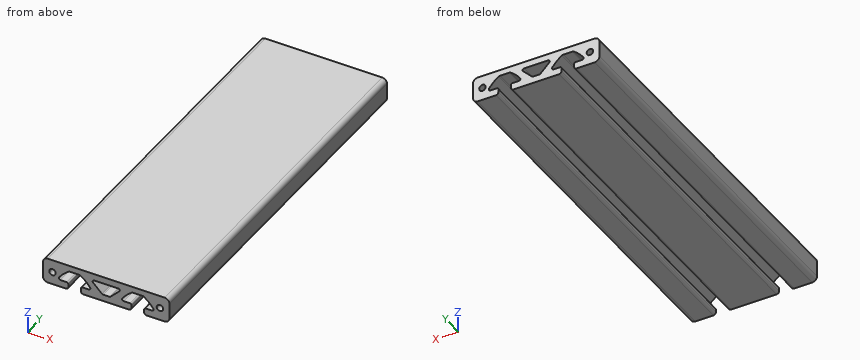
Autodesk Inventor part; units mm, degrees
ref_plane "Start Plane" through (0, 0, 0) normal (0, 1, 0) x (-1, 0, 0)
ref_plane "End Plane" through (0, 240, 0) normal (0, 1, 0) x (-1, 0, 0)
ref_plane "YZ Plane" through (0, 0, 0) normal (1, 0, 0) x (0, 1, 0)
ref_plane "Start Plane" through (0, 0, 0) normal (0, 1, 0) x (-1, 0, 0)
ref_plane "End Plane" through (0, 240, 0) normal (0, 1, 0) x (-1, 0, 0)
sketch "Sketch1" plane through (0, 0, 0) normal (0, 1, 0) x (-1, 0, 0)
  line L0 (40, -5) -> (40, 5)
  arc A0 (40, 5) -> (37, 8) centre (37, 5) ccw
  line L1 (37, 8) -> (-37, 8)
  line L2 (14.5, -8) -> (-14.5, -8)
  arc A1 (14.5, -8) -> (16, -6.5) centre (14.5, -6.5) ccw
  line L3 (-25.5, -8) -> (-37, -8)
  arc A2 (-25.5, -8) -> (-24, -6.5) centre (-25.5, -6.5) ccw
  arc A3 (-37, 8) -> (-40, 5) centre (-37, 5) ccw
  line L4 (-40, 5) -> (-40, -5)
  arc A4 (-40, -5) -> (-37, -8) centre (-37, -5) ccw
  line L5 (-24, -6.5) -> (-24, -4.5)
  arc A5 (-24, -4.5) -> (-25, -3.5) centre (-25, -4.5) ccw
  line L6 (-25, -3.5) -> (-29.0014, -3.5)
  arc A6 (-29.8106, -1.9125) -> (-29.0014, -3.5) centre (-29.0014, -2.5) ccw
  arc A7 (-23.7664, 3.9851) -> (-29.8106, -1.9125) centre (-9.58, -16.6) ccw
  arc A8 (-22.9152, 4.25) -> (-23.7664, 3.9851) centre (-22.9152, 2.75) ccw
  line L7 (-22.9152, 4.25) -> (-17.0848, 4.25)
  arc A9 (-16.2336, 3.9851) -> (-17.0848, 4.25) centre (-17.0848, 2.75) ccw
  arc A10 (-10.1894, -1.9125) -> (-16.2336, 3.9851) centre (-30.42, -16.6) ccw
  arc A11 (-10.9986, -3.5) -> (-10.1894, -1.9125) centre (-10.9986, -2.5) ccw
  line L8 (-10.9986, -3.5) -> (-15, -3.5)
  arc A12 (-15, -3.5) -> (-16, -4.5) centre (-15, -4.5) ccw
  line L9 (-16, -4.5) -> (-16, -6.5)
  arc A13 (-16, -6.5) -> (-14.5, -8) centre (-14.5, -6.5) ccw
  line L10 (16, -6.5) -> (16, -4.5)
  arc A14 (16, -4.5) -> (15, -3.5) centre (15, -4.5) ccw
  line L11 (15, -3.5) -> (10.9986, -3.5)
  arc A15 (10.1894, -1.9125) -> (10.9986, -3.5) centre (10.9986, -2.5) ccw
  arc A16 (16.2336, 3.9851) -> (10.1894, -1.9125) centre (30.42, -16.6) ccw
  arc A17 (17.0848, 4.25) -> (16.2336, 3.9851) centre (17.0848, 2.75) ccw
  line L12 (17.0848, 4.25) -> (22.9152, 4.25)
  arc A18 (23.7664, 3.9851) -> (22.9152, 4.25) centre (22.9152, 2.75) ccw
  arc A19 (29.8106, -1.9125) -> (23.7664, 3.9851) centre (9.58, -16.6) ccw
  arc A20 (29.0014, -3.5) -> (29.8106, -1.9125) centre (29.0014, -2.5) ccw
  line L13 (29.0014, -3.5) -> (25, -3.5)
  arc A21 (25, -3.5) -> (24, -4.5) centre (25, -4.5) ccw
  line L14 (1.9858, -3.8) -> (-1.9858, -3.8)
  arc A22 (-2.6929, -3.5071) -> (-1.9858, -3.8) centre (-1.9858, -2.8) ccw
  line L15 (-2.6929, -3.5071) -> (-8.2929, 2.0929)
  arc A23 (-7.5858, 3.8) -> (-8.2929, 2.0929) centre (-7.5858, 2.8) ccw
  line L16 (-7.5858, 3.8) -> (7.5858, 3.8)
  arc A24 (8.2929, 2.0929) -> (7.5858, 3.8) centre (7.5858, 2.8) ccw
  line L17 (8.2929, 2.0929) -> (2.6929, -3.5071)
  arc A25 (1.9858, -3.8) -> (2.6929, -3.5071) centre (1.9858, -2.8) ccw
  circle A26 centre (-34, 0) radius 2.05
  circle A27 centre (34, 0) radius 2.05
  line L18 (25.5, -8) -> (37, -8)
  arc A28 (24, -6.5) -> (25.5, -8) centre (25.5, -6.5) ccw
  arc A29 (37, -8) -> (40, -5) centre (37, -5) ccw
  line L19 (24, -6.5) -> (24, -4.5)
  point P0 (0, 0)
extrude "Body" add sketch "Sketch1" along normal up to surface (240 mm away) from surface at 0
sketch "Sketch2" plane through (0, 0, 0) normal (0, 1, 0) x (-1, 0, 0)
  line L0 (0, 0) -> (10, 0)
ref_plane "Work Plane3" through (0, 0, 0) normal (0, 0, -1) x (-1, 0, 0)
sketch "Sketch3" plane through (0, 0, 0) normal (0, 0, -1) x (-1, 0, 0)
  line L0 (-2, 0) -> (12, 0)
  line L1 (-2, 240) -> (12, 240)
  dimension "d15" = 240
sketch "Schizzo4" plane through (22.9152, 240, 4.25) normal (0, 0, -1) x (-1, 0, 0)
  point P0 (22.9152, -240)
equation "\"G_OFFSET_START\" = 0"
equation "\"G_OFFSET_END\" = 0"
equation "\"G_L\" = d15"
properties part number "10-081"
For this review, take the finished solid that the model builds, in its own axes (mm). Coordinates: 2 decimals unless noted, no trailing zeros. Order: outer loops, then holes, each group sorted by start corner. A loop starts at its lowest first (then second) coordinate and runs counter-clockwise, first axis right, second up. Notation, with made-up numbers: (-24.5, 5) -> (1.5, 5) arc R24 ccw to (1.5, 17) -> close; hole circle Ø7 at (16, 65). An arc over 180 degrees is marked (long way). Use CSV: the item, a comma, the result in double quotes. Start each with the question number.
Item 1: We need section B-B, the plane y = 131. Give the number of separate pieces and of enclosed holes in the cut face, then the cut area to 3 significant figures.
Item 2: We need section A-A, the plane x = -34. Give the boundary of the cut face in (y, z), then the cut area to 3 significant figures.
Item 3: Wall thickness on probe 1 along X at (y, z) = (190, -4.25); probe 2 along X at (y, z) = (137, 4); probe 3 along X at (y, z) = (197.5, 2.25): over which ranges is each line inside the solid? List them lowest first.
Item 4: Insertion check: pin 1 (1 mm diameter, centred on x = 17.5, z = -6, fed in from +Y); pin 2 (6.5 mm diameter, centred on x = -19, y = 81.5, fed in from -Z). Each pin has a flat end and moves straight along its axis. Give the tip position at first contact, or say it passes through.
Derived:
1,separate pieces,"1"
1,enclosed holes,"3"
1,area,"845 mm^2"
2,outline,"(0, -8) -> (240, -8) -> (240, -2.05) -> (0, -2.05) -> close; (0, 2.05) -> (240, 2.05) -> (240, 8) -> (0, 8) -> close"
2,area,"2,860 mm^2"
3,probe 1,"x = -40 to -24.03, -15.97 to 15.97, 24.03 to 40"
3,probe 2,"x = -40 to -23.74, -16.26 to 16.26, 23.74 to 40"
3,probe 3,"x = -40 to -26, -14 to -8.42, 8.42 to 14, 26 to 40"
4,pin 1,"passes through"
4,pin 2,"stops at z = -7.33"
